Geometry: final body of the model. Coordinates: model frame, mm. Face numbers are marked on the shaded views. Give positions to 0.01 mm unless a question says otherwise; leave off trailing zeros. Order: outer loops, then holes, each group sorted by start corner. A loop starts at its lowest first (then second) coordinate and runs counter-clockwise, first axis right, second up. Notation, with made-up numbers: (46.5, 41) - (81.5, 41) arc R29 cw to (81.5, 73) - close; hole circle Ø9 at (-23, 63.25). An arc over 180 degrees is marked (long way). One line per item, written item: value.
```python
from build123d import *

# Parameters (mm, degrees)
F2_R           = 5
F4_R           = 2.5
F5_DEPTH       = 25.001
F6_D           = 5
F6_CBORE_D     = 10
F6_CBORE_DEPTH = 4


# Not quite as in the source:
# - a fillet or chamfer that OpenCascade refuses, or shapes differently, is made with other operations: its cross-section is extruded or revolved along the edge and cut away or added


with BuildPart() as f1:
    # F0 (on Front) → F1 (revolve)
    with BuildSketch(Plane.XZ):
        with BuildLine():
            Line((0, 25), (0, 0))
            Line((0, 0), (14.5, 0))
            ThreePointArc((14.5, 0), (14.8535533906, 0.1464466094), (15, 0.5))
            Line((15, 0.5), (15, 3))
            ThreePointArc((15, 3), (14.4142135624, 4.4142135624), (13, 5))
            Line((13, 5), (8, 5))
            Line((8, 5), (8, 10))
            Line((8, 10), (15, 20))
            Line((15, 20), (15, 23))
            ThreePointArc((15, 23), (14.4142135624, 24.4142135624), (13, 25))
            Line((13, 25), (0, 25))
        make_face()
    revolve(axis=Axis((0, 0, 12.5), (0, 0, -1)))

    # F2
    f2_edges = [f1.edges().sort_by_distance(p)[0] for p in [
        (-8, 0, 10),
        (-15, 0, 20),
        (11.5, 0, 15),
    ]]
    fillet(f2_edges, radius=F2_R)

    # F3: fillet of radius 5 on 3 edges, made by hand

    # F3_s1 → F3_t2 (revolve)
    with BuildSketch(Plane.XZ):
        with BuildLine():
            ThreePointArc((7.9999979579, 8.4238888459), (9.8193871029, 5.9453387459), (12.7450873806, 5))
            Line((12.7450873806, 5), (8, 5))
            Line((8, 5), (7.9999979579, 8.4238888459))
        make_face()
    revolve(axis=Axis((0, 0, 5), (0, 0, -1)))

    # F4 (on face) → F5 (cut, through all)
    with BuildSketch(Plane.XY.offset(25)):
        Circle(F4_R)
    extrude(amount=-F5_DEPTH, mode=Mode.SUBTRACT)

    # F6 (through all)
    with Locations(Plane.XY.offset(25)):
        with Locations((0, 0)):
            CounterBoreHole(F6_D / 2, F6_CBORE_D / 2, F6_CBORE_DEPTH)


solid = f1.part
```
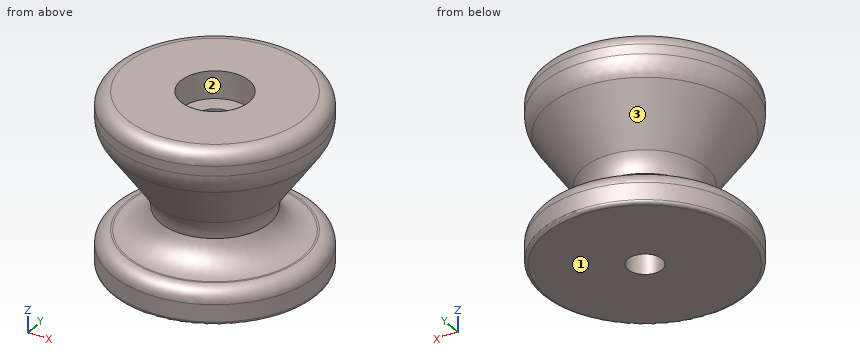
1) Mould query, pull axis Y, two halves, no side actions, for the marked faces 1, 2 and 3. Classes: released by +Y, released by -Y, zero draft, split by the parting line, or undercut.
Answers below:
face 1: zero draft
face 2: undercut
face 3: split by the parting line
2) Section A-A, the plane z = 16.5. Return loops of the section in (x, y), then the cut area to 3 significant figures.
Answers below:
outline: circle Ø25.1 at (0, 0); hole circle Ø5 at (0, 0)
area: 475 mm^2
3) Section B-B, the plane z = 7.5. Return loops of the section in (x, y).
Answers below:
outline: circle Ø16.83 at (0, 0); hole circle Ø5 at (0, 0)
4) Material intervals for line 1 along Y through (x, z) = (0, 22.4); line 2 along Y through (x, z) = (-2, 8.25); line 3 along Z through (x, y) = (10.5, -6), sorted ascending.
Answers below:
line 1: -15 to -5, 5 to 15
line 2: -7.81 to -1.5, 1.5 to 7.81
line 3: 0 to 5.04, 15.85 to 25
5) First-contact query: pin 1 (3 mm diameter, centred on x = -1.5, y = -1.5, fed in from +Z); pin 2 (1 mm diameter, centred on x = 10.5, y = 9, fed in from +Z); pin 3 (1 mm diameter, centred on x = -10.5, z = 9.5, fed in from +Y); pin 4 (2 mm diameter, centred on y = 6, z = 22, fed in from -X). Flat tips, straight axial feed; report the tip coordinate or a pass-through.
Answers below:
pin 1: z = 21
pin 2: z = 24.97
pin 3: through
pin 4: x = -14.14
